Could you check a few things on this model? Use its own coordinates, in mm. Face numbers are marked on the shaded views. A direction names the side the tool comes from. Coordinates: 2 decimals unless noted, no trailing zeros. Order: outer loops, then holes, each group sorted by start corner. A loop starts at its lowest first (then second) coordinate and runs counter-clockwise, first axis right, second up. Notation, with made-up numbers: (84, 55) - (128, 55) arc R29 cw to (128, 94) - close; hole circle Ø5 at (83, -12.5). An arc over 180 degrees is marked (long way). Answer as CSV lines item,"result". Start each with the question number.
1. I want a section at B-B, the plane y = 154.5. List the corners of the cut face in (x, z) for me (3 decimals).
2. I want a section at C-C, the plane z = 33.5. List the corners of the cut face in (x, y) for me.
3. I want a section at A-A, the plane y = 88.9. List the corners of the cut face in (x, z) for me (3 decimals), and give its area (3 significant figures).
4. For the marked faces 1, 2, 3 and 4, which set-ups out of +Z, -Z, +X, -X, +Y, -Y let a thin tool reach every point of the face, with its end or its side?
5. For pin 1 (3 mm diameter, centred on x = 522.5, y = 76.5, fed in from +Z); pin 2 (1 mm diameter, centred on x = 376, z = 123.5, fed in from +Y), each with a flat end and sliding along its axis, tell me the tip position at first contact or that it passes through.
6. I want a section at D-D, the plane y = 126. List the corners of the cut face in (x, z) for me (3 decimals), and give its area (3 significant figures).
7. I need wall thicknesses on probe 1 along Z at (x, y) = (392.5, 43) (3 decimals); probe 2 along X at (y, z) = (51.5, 106); probe 3 along X at (y, z) = (104.5, 72). Which ranges of each line are inside material? Lowest first, please.
8. Thinking about a two-plate mould opening in X: for the marked faces 5, 6, 7 and 8, which applies, released by +X, released by -X, zero draft, split by the parting line, or undercut?
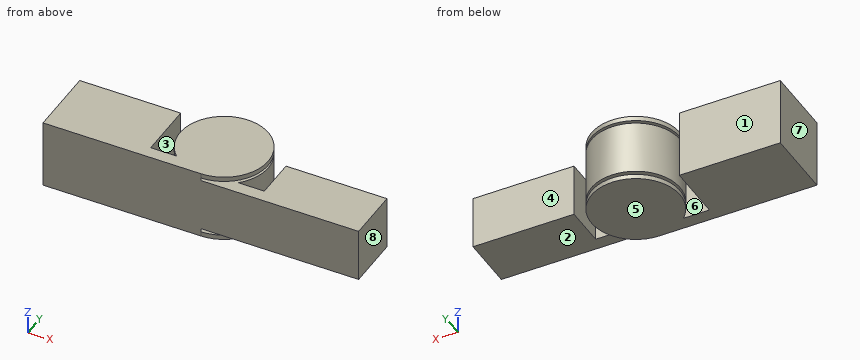
from build123d import *

# Parameters (mm, degrees)
BOSS_EXTRUDE1_DEPTH     = 139.7
SKETCH3_R               = 88.9
CUT_EXTRUDE1_DEPTH      = 60.325
CUT_EXTRUDE1_DEPTH_BACK = 60.325
BOSS_EXTRUDE2_START     = 16.51
BOSS_EXTRUDE2_DEPTH     = 107.95


with BuildPart() as part:
    # Sketch1 → Boss-Extrude1 (new body)
    with BuildSketch(Plane.XY):
        with BuildLine():
            Line((203.2, 0), (317.5, 0))
            ThreePointArc((317.5, 0), (351.101041651, 171.20540687), (255.282960533, 25.4))
            Line((255.282960533, 25.4), (203.2, 25.4))
            Line((203.2, 25.4), (203.2, 139.7))
            Line((203.2, 139.7), (0, 139.7))
            Line((0, 139.7), (0, 0))
            Line((0, 0), (203.2, 0))
        make_face()
    extrude(amount=BOSS_EXTRUDE1_DEPTH)

    # Sketch3 → Cut-Extrude1 (cut, two sides)
    with BuildSketch(Plane.XY.offset(69.85)) as cut_extrude1_sk:
        with Locations((317.5, 88.9)):
            Circle(SKETCH3_R)
    extrude(amount=CUT_EXTRUDE1_DEPTH, mode=Mode.SUBTRACT)
    extrude(cut_extrude1_sk.sketch, amount=-CUT_EXTRUDE1_DEPTH_BACK, mode=Mode.SUBTRACT)

    # Sketch2 → Boss-Extrude2 (add)
    with BuildSketch(Plane.XY.offset(BOSS_EXTRUDE2_START)):
        with BuildLine():
            Line((317.5, 0), (431.8, 0))
            Line((431.8, 0), (635, 0))
            Line((635, 0), (635, 107.95))
            Line((635, 107.95), (431.8, 107.95))
            Line((431.8, 107.95), (431.8, 25.4))
            Line((431.8, 25.4), (379.717039467, 25.4))
            ThreePointArc((379.717039467, 25.4), (283.898958349, 171.20540687), (317.5, 0))
        make_face()
    extrude(amount=BOSS_EXTRUDE2_DEPTH)


solid = part.part
Solved:
1,outline,"(257.501, 0) - (377.499, 0) - (377.499, 9.525) - (257.501, 9.525) - close; (257.501, 16.51) - (377.499, 16.51) - (377.499, 124.46) - (257.501, 124.46) - close; (257.501, 130.175) - (377.499, 130.175) - (377.499, 139.7) - (257.501, 139.7) - close"
2,outline,"(0, 0) - (635, 0) - (635, 107.95) - (431.8, 107.95) - (431.8, 25.4) - (379.72, 25.4) arc R88.9 ccw (long way) to (255.28, 25.4) - (203.2, 25.4) - (203.2, 139.7) - (0, 139.7) - close"
3,outline,"(0, 0) - (203.2, 0) - (203.2, 139.7) - (0, 139.7) - close; (228.6, 0) - (406.4, 0) - (406.4, 9.525) - (228.6, 9.525) - close; (228.6, 16.51) - (406.4, 16.51) - (406.4, 124.46) - (228.6, 124.46) - close; (228.6, 130.175) - (406.4, 130.175) - (406.4, 139.7) - (228.6, 139.7) - close; (431.8, 16.51) - (635, 16.51) - (635, 124.46) - (431.8, 124.46) - close"
3,area,"72,900 mm2"
4,face 1,"+Z, -Z, -X, +Y"
4,face 2,"+X, +Y"
4,face 3,"+Z, -Z, +Y"
4,face 4,"+Z, -Z, +X, +Y"
5,pin 1,"stops at z = 124.46"
5,pin 2,"stops at y = 156.27"
6,outline,"(0, 0) - (203.2, 0) - (203.2, 139.7) - (0, 139.7) - close; (236.711, 0) - (398.289, 0) - (398.289, 9.525) - (236.711, 9.525) - close; (236.711, 16.51) - (398.289, 16.51) - (398.289, 124.46) - (236.711, 124.46) - close; (236.711, 130.175) - (398.289, 130.175) - (398.289, 139.7) - (236.711, 139.7) - close"
6,area,"48,900 mm2"
7,probe 1,"z = 0 to 9.525, 16.51 to 124.46, 130.175 to 139.7"
7,probe 2,"x = 0 to 203.2, 236.85 to 398.15, 431.8 to 635"
7,probe 3,"x = 0 to 203.2, 229.98 to 405.02, 431.8 to 635"
8,face 5,"zero draft"
8,face 6,"undercut"
8,face 7,"released by -X"
8,face 8,"released by +X"
